Read the model definition and answer for the solid it produces. Units are mm, in the model's axes. A direction names the side the tool comes from. Give positions to 0.01 mm unless a question says otherwise; leave off trailing zeros. Write each loop counter-clockwise with the first axis right and the second up, starting at its lowest first coordinate (ties: lowest second). Pieces come first, ordered by that corner, then holes. Notation, with made-up numbers: M 27,60.25 L 40,60.25 A17 cw 40,67.25 Z; hole C 71.25,-35.75 d6. An arc over 180 degrees is marked long. Use a Markdown table: item, result. Add a question column.
Item 1: A cutting plane is placed at B-B on y = -10.5. Determine the outline of the cut face in (x, z).
Item 2: Consider probe 1 along X at (y, z) = (25.5, 16); probe 2 along Z at (x, y) = (19.5, 0.5). Determine where each line is inside the solid, lowest interval first. Write a range as [from, to].
Item 3: For faces 1 (the flat face through (-1, -1, 25.4)), 2 (the flat face through (-1, 1, 101.6)), determine the directions among +Z, -Z, +X, -X, +Y, -Y from which every point of the face is accessible in a straight line to the end or side of a thin tool.
Item 4: A cutting plane is placed at C-C on x = 23. Determine the outline of the cut face in (y, z), then the cut area to 3 significant figures.
Item 5: The mould has two halves that part along X. Classify faces 3 (the flat face through (-50, 1, 0)), 4 (the flat face through (-36.855, -1, 13)), 5 (the flat face through (36.855, -1, 13)), 6 (the flat face through (-63.5, -1, 50)): pulls with the +X half, pulls with the -X half, needs draft (parallel to the pull), parting line crosses it, or undercut.
Item 6: Given P1, Ø5, axis at x = 4.5, y = 52.5, coming from the -Z side, flat-ended and moving along its own axis, determine where the tip first touches the part or whether it passes through.
Item 7: A cutting plane is placed at A-A on z = 9.5. Determine the outline of the cut face in (x, y), then the cut area to 3 significant figures.
from build123d import *

# Parameters (mm, degrees)
F0_W     = 127
F0_H     = 152.4
F1_DEPTH = 101.6
F2_W     = 73.71036
F2_H     = 50.8
F3_DEPTH = 2540


with BuildPart() as f1:
    # F0 (on Top) → F1 (new body)
    with BuildSketch(Plane.XY):
        Rectangle(F0_W, F0_H)
    extrude(amount=F1_DEPTH)

    # F2 (on Front) → F3 (cut, symmetric)
    with BuildSketch(Plane.XZ):
        Rectangle(F2_W, F2_H)
    extrude(amount=F3_DEPTH, both=True, mode=Mode.SUBTRACT)


solid = f1.part
Filled in:
| question | item | result |
|---|---|---|
| 1 | outline | M -63.5,0 L -36.86,0 L -36.86,25.4 L 36.86,25.4 L 36.86,0 L 63.5,0 L 63.5,101.6 L -63.5,101.6 Z |
| 2 | probe 1 | [-63.5, -36.86], [36.86, 63.5] |
| 2 | probe 2 | [25.4, 101.6] |
| 3 | face 1 | -Z, +Y, -Y |
| 3 | face 2 | +Z, +X, -X, +Y, -Y |
| 4 | outline | M -76.2,25.4 L 76.2,25.4 L 76.2,101.6 L -76.2,101.6 Z |
| 4 | area | 11,600 mm² |
| 5 | face 3 | needs draft |
| 5 | face 4 | undercut |
| 5 | face 5 | undercut |
| 5 | face 6 | pulls with the -X half |
| 6 | P1 | z = 25.4 |
| 7 | outline | M -63.5,-76.2 L -36.86,-76.2 L -36.86,76.2 L -63.5,76.2 Z; M 36.86,-76.2 L 63.5,-76.2 L 63.5,76.2 L 36.86,76.2 Z |
| 7 | area | 8,120 mm² |
